CAD build for the part. Positions are in the model's coordinates, mm. Face numbers are marked on the shaded views. Round coordinates to 2 decimals unless told otherwise and drop trailing zeros. Loops run counter-clockwise (first coordinate to the right, second up) from the corner with the lowest first, then second, coordinate; pieces in that order, holes last.
from build123d import *

# Parameters (mm, degrees)
SKETCH_1_W      = 87.739735524
SKETCH_1_H      = 68.368625084
SKETCH_1_R      = 26
EXTRUDE_1_DEPTH = 80


with BuildPart() as part:
    # 草图1 → 凸台-拉伸1 (new body)
    with BuildSketch(Plane.XY):
        with Locations((-1.63708593, -0.456202936)):
            Rectangle(SKETCH_1_W, SKETCH_1_H)
        with Locations((-1.63708593, 0)):
            Circle(SKETCH_1_R, mode=Mode.SUBTRACT)
    extrude(amount=EXTRUDE_1_DEPTH)


solid = part.part
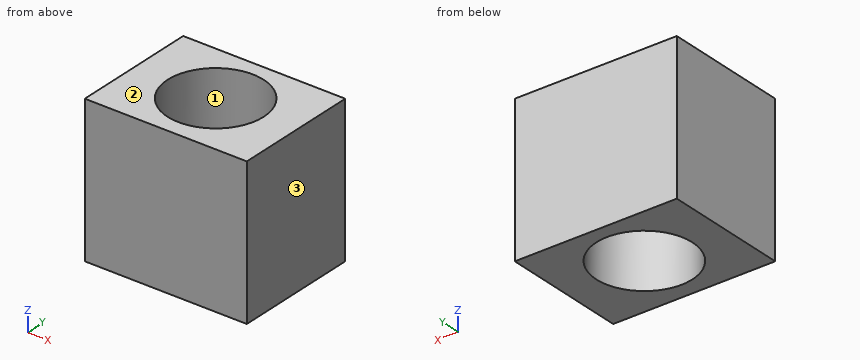
Item 1: Cut at C-C (z = 6.5). List the corners of the cut face in (x, y), plus the area to 3 significant figures.
Verdict:
outline: (-45.51, -34.64) - (42.23, -34.64) - (42.23, 33.73) - (-45.51, 33.73) - close; hole circle Ø52 at (-1.64, 0)
area: 3,870 mm2
Item 2: Cut at B-B (x = -12). List the corners of the cut face in (y, z).
Verdict:
outline: (-34.64, 0) - (-23.85, 0) - (-23.85, 80) - (-34.64, 80) - close; (23.85, 0) - (33.73, 0) - (33.73, 80) - (23.85, 80) - close
Item 3: Wall check: L1, parallel to X at y = 21, z = 18; L2, parallel to Y at x = 2.5, z = 44; L3, parallel to X at y = -11.5, z = 58.5. Give the ranges that are in metal, low to high.
Verdict:
L1: x = -45.51 to -16.97, 13.69 to 42.23
L2: y = -34.64 to -25.67, 25.67 to 33.73
L3: x = -45.51 to -24.96, 21.68 to 42.23
Item 4: Mould opens along X. For the marked faces 1, 2 and 3 say: released by +X, released by -X, zero draft, split by the parting line, or undercut.
Verdict:
face 1: undercut
face 2: zero draft
face 3: released by +X
Item 5: Cut at A-A (y = 0). List the corners of the cut face in (x, z).
Verdict:
outline: (-45.51, 0) - (-27.64, 0) - (-27.64, 80) - (-45.51, 80) - close; (24.36, 0) - (42.23, 0) - (42.23, 80) - (24.36, 80) - close
